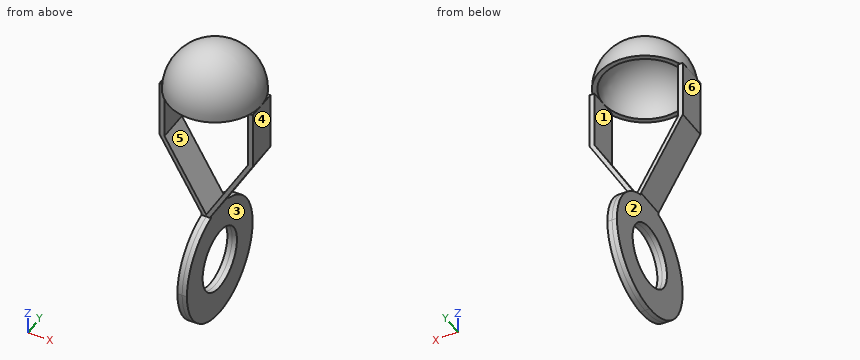
from build123d import *
from build123d.topology import SkipClean

# Parameters (mm, degrees)
BOSS_EXTRUDE1_DEPTH = 4.7625
SKETCH2_R           = 2.4892
SKETCH2_W           = 10.40972438
SKETCH2_H           = 3.4925
CUT_EXTRUDE1_DEPTH  = 12.922988592


# Read off the part's stored shape, not the designer's step: Revolve2
with BuildPart() as part:
    # Sketch1 → Boss-Extrude1 (new, symmetric)
    with BuildSketch(Plane(origin=(0, 0, 0), x_dir=(1, 0, 0), z_dir=(0, 1, 0))):
        Polygon((0, 0), (3.33375, -5.77422438), (3.33375, -10.40972438), (3.71475, -10.40972438), (3.71475, -5.77422438), (0.381, 0), (0.381, 9.525), (0, 9.525), align=None)
    boss_extrude1 = extrude(amount=BOSS_EXTRUDE1_DEPTH, both=True)

    # Sketch2 → Cut-Extrude1 (cut, symmetric)
    with BuildSketch(Plane(origin=(0.381, 0, 0), x_dir=(0, 0, -1), z_dir=(1, 0, 0))):
        with BuildLine():
            Line((0.172455746, -1.27), (0, -1.27))
            Line((0, -1.27), (0, -4.7625))
            Line((0, -4.7625), (4.7625, -4.7625))
            ThreePointArc((4.7625, -4.7625), (1.878663038, -3.790104303), (0.172455746, -1.27))
        make_face()
        with BuildLine():
            ThreePointArc((9.525, 0), (8.130096045, -3.367596045), (4.7625, -4.7625))
            Line((4.7625, -4.7625), (9.525, -4.7625))
            Line((9.525, -4.7625), (9.525, 0))
        make_face()
        with BuildLine():
            ThreePointArc((4.762500002, 4.7625), (8.130096046, 3.367596045), (9.525, 0))
            Line((9.525, 0), (9.525, 4.7625))
            Line((9.525, 4.7625), (4.762500002, 4.7625))
        make_face()
        with BuildLine():
            Line((0, 4.7625), (0, 1.27))
            Line((0, 1.27), (0.172455746, 1.27))
            ThreePointArc((0.172455746, 1.27), (1.878663039, 3.790104303), (4.762500002, 4.7625))
            Line((4.762500002, 4.7625), (0, 4.7625))
        make_face()
        with Locations((4.7625, 0)):
            Circle(SKETCH2_R)
        with Locations((-5.20486219, 3.01625)):
            Rectangle(SKETCH2_W, SKETCH2_H)
        with Locations((-5.20486219, -3.01625)):
            Rectangle(SKETCH2_W, SKETCH2_H)
    cut_extrude1 = extrude(amount=CUT_EXTRUDE1_DEPTH, both=True, mode=Mode.SUBTRACT)

    # Mirror1: Boss-Extrude1, Cut-Extrude1 across plane
    with SkipClean():  # the faces are left unmerged after this step: merging them gives an invalid solid
        add(boss_extrude1.mirror(Plane(origin=(0, 0, 0), x_dir=(0, 0, 1), z_dir=(1, 0, 0))))
        add(cut_extrude1.mirror(Plane(origin=(0, 0, 0), x_dir=(0, 0, 1), z_dir=(1, 0, 0))), mode=Mode.SUBTRACT)

    # Revolve2 outline → Revolve2 (revolve)
    with SkipClean():  # the faces are left unmerged after this step: merging them gives an invalid solid
        with BuildSketch(Plane.XZ):
            with BuildLine():
                ThreePointArc((0, 13.74347438), (2.357317233, 12.76704161), (3.33375, 10.409724376))
                Line((3.33375, 10.409724376), (3.71475, 10.409724377))
                ThreePointArc((3.71475, 10.409724377), (2.626724917, 13.036449294), (0, 14.12447438))
                Line((0, 14.12447438), (0, 13.74347438))
            make_face()
        revolve(axis=Axis((0, 0, 0), (0, 0, 1)))


solid = part.part
Build history of the part. All positions in model axes, mm. Face numbers are marked on the shaded views. A direction names the side the tool comes from. Round coordinates to 2 decimals unless told otherwise and drop trailing zeros. Write each loop counter-clockwise with the first axis right and the second up, starting at its lowest first coordinate (ties: lowest second). Pieces come first, ordered by that corner, then holes. Notation, with made-up numbers: (86.25, 84) - (129.25, 84) arc R22 ccw to (129.25, 94) - close; hole circle Ø5 at (12.25, 34). An arc over 180 degrees is marked (long way). Use CSV: the item, a comma, the result in double quotes.
(1) Band-saw the part on D-D (y = -0.75). Write the cut outline in (x, z), plus the area to 3 significant figures.
Response:
outline,"(-3.71, 5.77) - (-0.38, 0) - (-0.38, -2.39) - (0.38, -2.39) - (0.38, 0) - (3.71, 5.77) - (3.71, 10.41) - (3.64, 10.41) arc R3.64 ccw to (-3.64, 10.41) - (-3.71, 10.41) - close; (-0.38, -9.47) - (0.38, -9.47) - (0.38, -7.14) - (-0.38, -7.14) - close; hole (-3.33, 5.77) - (0, 0) - (3.33, 5.77) - (3.33, 10.41) - (3.25, 10.41) arc R3.25 ccw to (-3.25, 10.41) - (-3.33, 10.41) - close"
area,"15.7 mm²"
(2) Wall check: line 1 (X direction, y = 0.75, z = -1); line 2 (Z direction, x = -0.2, y = 0) (3 decimals); line 3 (Z direction, x = -1.25, y = -1). Give the ranges that are in metal, low to high.
Response:
line 1,"-0.38 to 0.38"
line 2,"-9.525 to -7.252, -2.273 to 0.346, 13.737 to 14.119"
line 3,"1.51 to 2.17, 13.33 to 13.76"
(3) Band-saw the part on A-A (y = 1). Write the cut outline in (x, z).
Response:
outline,"(-3.71, 5.77) - (-0.38, 0) - (-0.38, -2.48) - (0.38, -2.48) - (0.38, 0) - (3.71, 5.77) - (3.71, 10.41) - (3.58, 10.41) arc R3.58 ccw to (-3.58, 10.41) - (-3.71, 10.41) - close; (-0.38, -9.42) - (0.38, -9.42) - (0.38, -7.04) - (-0.38, -7.04) - close; hole (-3.33, 5.77) - (0, 0) - (3.33, 5.77) - (3.33, 10.41) - (3.18, 10.41) arc R3.18 ccw to (-3.18, 10.41) - (-3.33, 10.41) - close"
(4) Pin check, flat tips, straight feed: P1, Ø1.5, axis at x = -1, y = 0.5, coming from the +Z side; P2, Ø4, axis at y = 0, z = -4.76, coming from the -X side; P3, Ø1.1, axis at x = 0.5, y = 2.5, coming from the -Z side; P4, Ø2, axis at x = 2, z = 1.5, coming from the +Y side. Stop position of each tip, or through.
Response:
P1,"z = 14.11"
P2,"through"
P3,"z = -9.1"
P4,"y = 1.27"
(5) 3-axis set-ups, long thin cutter, end or side, ignore diameter. For the marked faces 1, 2 and 3: which of +Z, -Z, +X, -X, +Y, -Y reach the whole face in a straight line?
Response:
face 1,"+Y, -Y"
face 2,"-Z, -X, +Y, -Y"
face 3,"-Z, +X, +Y, -Y"
(6) Band-saw the part on B-B (z = -5.5). Write the cut outline in (x, y).
Response:
outline,"(-0.38, -4.71) - (0.38, -4.71) - (0.38, -2.38) - (-0.38, -2.38) - close; (-0.38, 2.38) - (0.38, 2.38) - (0.38, 4.71) - (-0.38, 4.71) - close"
(7) Mould opens along X. For the marked faces 4, 5 and 6 say: pulls with the +X half, pulls with the -X half, needs draft (parallel to the pull), parting line crosses it, or undercut.
Response:
face 4,"pulls with the +X half"
face 5,"undercut"
face 6,"pulls with the -X half"
(8) Band-saw the part on C-C (x = -0.75). Write the cut outline in (y, z).
Response:
outline,"(-3.64, 10.41) - (-3.25, 10.41) arc R3.25 cw to (3.25, 10.41) - (3.64, 10.41) arc R3.64 ccw to start; (-1.27, 0.64) - (1.27, 0.64) - (1.27, 1.3) - (-1.27, 1.3) - close"
